```python
from build123d import *

# Parameters (mm, degrees)
SKETCH_1_W               = 24
SKETCH_1_H               = 38
EXTRUDE_1_DEPTH          = 5
SKETCH_2_R               = 2.75
CUT_EXTRUDE_1_DEPTH      = 10.25
CUT_EXTRUDE_2_DEPTH      = 24.021728866
CUT_EXTRUDE_2_DEPTH_BACK = 24.021728866
SKETCH_3_R               = 1
CUT_EXTRUDE_3_DEPTH      = 0.5
SKETCH_5_R               = 1.75
CUT_EXTRUDE_4_DEPTH      = 24.021728866
FILLET_1_R               = 3
FILLET_2_R               = 3
SKETCH_6_R               = 1.5
CUT_EXTRUDE_5_DEPTH      = 8
FILLET_3_R               = 0.5
SKETCH_7_R               = 1.25
CUT_EXTRUDE_6_DEPTH      = 24.02172894
SKETCH_8_R               = 3
CUT_EXTRUDE_7_DEPTH      = 2
CUT_EXTRUDE_8_DEPTH      = 2
FILLET_4_R               = 0.5


with BuildPart() as part:
    # Эскиз1 → Бобышка-Вытянуть1 (new body)
    with BuildSketch(Plane(origin=(0, 0, 0), x_dir=(1, 0, 0), z_dir=(0, 1, 0))):
        Rectangle(SKETCH_1_W, SKETCH_1_H)
    extrude(amount=EXTRUDE_1_DEPTH)

    # Эскиз2 → Вырез-Вытянуть1 (cut, symmetric)
    with BuildSketch(Plane(origin=(0, 0, 0), x_dir=(0, 0, -1), z_dir=(1, 0, 0))):
        with Locations((-12.75, 5)):
            Circle(SKETCH_2_R)
        with Locations((12.75, 5)):
            Circle(SKETCH_2_R)
    extrude(amount=CUT_EXTRUDE_1_DEPTH, both=True, mode=Mode.SUBTRACT)

    # Эскиз3 → Вырез-Вытянуть2 (cut, two sides: drawn at the far end of the back side and taken through both)
    with BuildSketch(Plane(origin=(0, 0, 0), x_dir=(0, 0, -1), z_dir=(1, 0, 0)).offset(-CUT_EXTRUDE_2_DEPTH_BACK)):
        with Locations((-12.75, 5)):
            Circle(SKETCH_3_R)
        with Locations((12.75, 5)):
            Circle(SKETCH_3_R)
    extrude(amount=CUT_EXTRUDE_2_DEPTH + CUT_EXTRUDE_2_DEPTH_BACK, mode=Mode.SUBTRACT)

    # Эскиз4 → Вырез-Вытянуть3 (cut)
    with BuildSketch(Plane(origin=(0, 5, 0), x_dir=(1, 0, 0), z_dir=(0, 1, 0))):
        with BuildLine():
            Line((4, 7), (-12, 7))
            Line((-12, 7), (-12, 5.5))
            Line((-12, 5.5), (-0.330127019, 5.5))
            ThreePointArc((-0.330127019, 5.5), (-3, 0), (-0.330127019, -5.5))
            Line((-0.330127019, -5.5), (-12, -5.5))
            Line((-12, -5.5), (-12, -7))
            Line((-12, -7), (4, -7))
            ThreePointArc((4, -7), (8.677071733, -5.208166664), (10.959705454, -0.75))
            Line((10.959705454, -0.75), (12, -0.75))
            Line((12, -0.75), (12, 0.75))
            Line((12, 0.75), (10.959705454, 0.75))
            ThreePointArc((10.959705454, 0.75), (8.677071733, 5.208166664), (4, 7))
        make_face()
    extrude(amount=-CUT_EXTRUDE_3_DEPTH, mode=Mode.SUBTRACT)

    # Эскиз5 → Вырез-Вытянуть4 (cut, through all)
    with BuildSketch(Plane(origin=(0, 5, 0), x_dir=(1, 0, 0), z_dir=(0, 1, 0))):
        with Locations(Location((4, 0, 0), (0, 0, 270))):
            Circle(SKETCH_5_R)
        with Locations(Location((-7, 0, 0), (0, 0, 270))):
            Circle(SKETCH_5_R)
    extrude(amount=-CUT_EXTRUDE_4_DEPTH, mode=Mode.SUBTRACT)

    # Скругление1
    fillet_1_edges = [part.edges().sort_by_distance(p)[0] for p in [
        (-0.330127019, 4.75, 5.5),
        (-0.330127019, 4.75, -5.5),
    ]]
    fillet(fillet_1_edges, radius=FILLET_1_R)

    # Скругление2
    fillet_2_edges = [part.edges().sort_by_distance(p)[0] for p in [
        (12, 2.5, 19),
        (-12, 2.5, 19),
        (-12, 2.5, -19),
        (12, 2.5, -19),
    ]]
    fillet(fillet_2_edges, radius=FILLET_2_R)

    # Эскиз6 → Вырез-Вытянуть5 (cut)
    with BuildSketch(Plane.ZY.offset(12)):
        with Locations((0, 5)):
            Circle(SKETCH_6_R)
    extrude(amount=-CUT_EXTRUDE_5_DEPTH, mode=Mode.SUBTRACT)

    # Скругление3
    fillet_3_edges = [part.edges().sort_by_distance(p)[0] for p in [
        (10.959705454, 4.75, -0.75),
        (10.959705454, 4.75, 0.75),
    ]]
    fillet(fillet_3_edges, radius=FILLET_3_R)

    # Эскиз7 → Вырез-Вытянуть6 (cut, through all)
    with BuildSketch(Plane(origin=(0, 5, 0), x_dir=(1, 0, 0), z_dir=(0, 1, 0))):
        with Locations(Location((-7, 17, 0), (0, 0, 270))):
            Circle(SKETCH_7_R)
        with Locations(Location((7, 17, 0), (0, 0, 270))):
            Circle(SKETCH_7_R)
        with Locations(Location((7, -17, 0), (0, 0, 270))):
            Circle(SKETCH_7_R)
        with Locations(Location((-7, -17, 0), (0, 0, 270))):
            Circle(SKETCH_7_R)
    extrude(amount=-CUT_EXTRUDE_6_DEPTH, mode=Mode.SUBTRACT)

    # Эскиз8 → Вырез-Вытянуть7 (cut)
    with BuildSketch(Plane.XZ):
        with Locations(Location((4, 0, 0), (0, 0, 270))):
            Circle(SKETCH_8_R)
        with Locations(Location((-7, 0, 0), (0, 0, 270))):
            Circle(SKETCH_8_R)
    extrude(amount=-CUT_EXTRUDE_7_DEPTH, mode=Mode.SUBTRACT)

    # Эскиз9 → Вырез-Вытянуть8 (cut)
    with BuildSketch(Plane.XZ):
        with BuildLine():
            Line((-9.05, 17), (-9.05, 20))
            Line((-9.05, 20), (-4.95, 20))
            Line((-4.95, 20), (-4.95, 17))
            ThreePointArc((-4.95, 17), (-7, 14.95), (-9.05, 17))
        make_face()
        with BuildLine():
            Line((9.05, 17), (9.05, 20))
            Line((9.05, 20), (4.95, 20))
            Line((4.95, 20), (4.95, 17))
            ThreePointArc((4.95, 17), (7, 14.95), (9.05, 17))
        make_face()
        with BuildLine():
            Line((4.95, -20), (4.95, -17))
            ThreePointArc((4.95, -17), (7, -14.95), (9.05, -17))
            Line((9.05, -17), (9.05, -20))
            Line((9.05, -20), (4.95, -20))
        make_face()
        with BuildLine():
            Line((-9.05, -17), (-9.05, -20))
            Line((-9.05, -20), (-4.95, -20))
            Line((-4.95, -20), (-4.95, -17))
            ThreePointArc((-4.95, -17), (-7, -14.95), (-9.05, -17))
        make_face()
    extrude(amount=-CUT_EXTRUDE_8_DEPTH, mode=Mode.SUBTRACT)

    # Скругление4
    fillet_4_edges = [part.edges().sort_by_distance(p)[0] for p in [
        (9.05, 1, 18.999583304),
        (-9.05, 1, 18.999583304),
        (9.05, 1, -18.999583304),
        (-9.05, 1, -18.999583304),
        (-4.95, 1, -19),
        (4.95, 1, -19),
        (4.95, 1, 19),
        (-4.95, 1, 19),
    ]]
    fillet(fillet_4_edges, radius=FILLET_4_R)


solid = part.part
```
Work out the finished part from the listing and answer in its coordinate system (mm). A direction names the side the tool comes from. Give positions to 0.01 mm unless a question says otherwise; leave off trailing zeros. Loops run counter-clockwise (first coordinate to the right, second up) from the corner with the lowest first, then second, coordinate; pieces in that order, holes last. Notation, with made-up numbers: (-4.5, -37) -> (23.5, -37) arc R29 cw to (23.5, -5) -> close; hole circle Ø6 at (16.25, 64.5). An arc over 180 degrees is marked (long way). One line per question, with ' | ' between items. Start each with the question number.
1) Each of these flat-tipped pins is pushed along its axis until it touches: pin 1 (1.6 mm diameter, centred on y = 1.5, z = 17.5, fed in from +X); pin 2 (1.2 mm diameter, centred on y = 0.5, z = 18, fed in from -X); pin 3 (1.6 mm diameter, centred on y = 1, z = 18, fed in from +X). Where does it stop, or does it pass through?
2) For faces 5 (the face through (-4, 4, 0)), 6 (the face through (8, 2, -18)), 7 (the face through (8.57, 4.75, -5.3)), 8 (the face through (9.05, 1, 18)), determine the directions among +Z, -Z, +X, -X, +Y, -Y from which every point of the face is accessible in a straight line to the end or side of a thin tool.
3) Straight lines are drawn through the part: L1, parallel to X at y = 2.95, z = -11; L2, parallel to X at y = 4.4, z = 0; L3, parallel to X at y = 0.65, z = 0. For each, find the intervals that lie inside material, in ascending order.
4) Determine the mould class of faces 1 (the face through (-12, 2, 0)), 2 (the face through (0, 0, 0)), 3 (the face through (2.29, 3.27, -0.38)), 4 (the face through (-6.95, 0.99, -14.95)) for opening direction X: +X half, -X half, draft (parallel to the pull), parting line (faces both ways), or undercut.
5) Section C-C, the plane x = -7 is taken. State how many separate pieces and enclosed holes the cut face has, then the cut area to 3 significant figures.
6) Section A-A, the plane z = 0 is taken. Determine the outline of the cut face in (x, y).
7) Section B-B, the plane x = 3 is taken. Determine the outline of the cut face in (y, z), then the cut area to 3 significant figures.
Resolved:
1) pin 1: x = 11.92 | pin 2: x = -11.65 | pin 3: x = 11.75
2) face 5: -X, +Y | face 6: -Z, -Y | face 7: +Y | face 8: +Z, -Y
3) L1: -12 to -10.25, 10.25 to 12 | L2: -4 to 2.25, 5.75 to 12 | L3: -12 to -10, -4 to 1, 7 to 12
4) face 1: -X half | face 2: draft | face 3: undercut | face 4: undercut
5) separate pieces: 4 | enclosed holes: 0 | area: 111 mm2
6) outline: (-12, 0) -> (-10, 0) -> (-10, 2) -> (-8.75, 2) -> (-8.75, 3.5) -> (-12, 3.5) -> close; (-5.25, 2) -> (-4, 2) -> (-4, 0) -> (1, 0) -> (1, 2) -> (2.25, 2) -> (2.25, 4.5) -> (-3, 4.5) -> (-3, 5) -> (-4, 5) -> (-4, 3.5) -> (-5.25, 3.5) -> close; (5.75, 2) -> (7, 2) -> (7, 0) -> (12, 0) -> (12, 4.5) -> (5.75, 4.5) -> close
7) outline: (0, -19) -> (5, -19) -> (5, -15.5) arc R2.75 cw to (5, -10) -> (5, -7) -> (4.5, -7) -> (4.5, -1.44) -> (2, -1.44) -> (2, -2.83) -> (0, -2.83) -> close; (0, 2.83) -> (2, 2.83) -> (2, 1.44) -> (4.5, 1.44) -> (4.5, 7) -> (5, 7) -> (5, 10) arc R2.75 cw to (5, 15.5) -> (5, 19) -> (0, 19) -> close | area: 141 mm2
